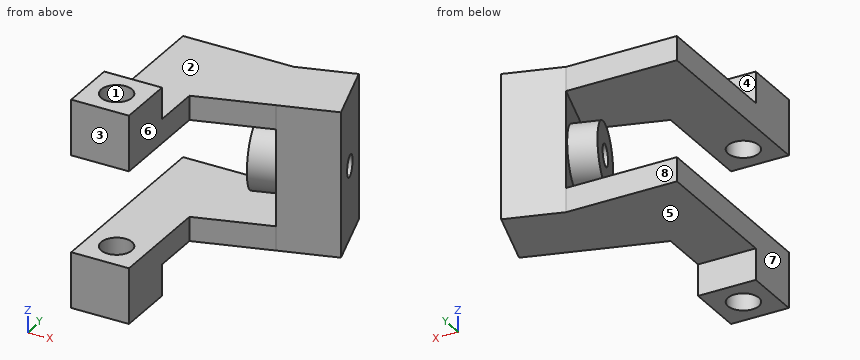
from build123d import *

# Parameters (mm, degrees)
BOSS_EXTRUDE1_DEPTH     = 9.525
SKETCH2_W               = 12.7
SKETCH2_H               = 25.806397913
CUT_EXTRUDE1_DEPTH      = 14.822389654
CUT_EXTRUDE1_DEPTH_BACK = 4.513666667
SKETCH3_W               = 19.05
SKETCH3_H               = 9.271
SKETCH3_R               = 1.397
BOSS_EXTRUDE2_DEPTH     = 7.62
SKETCH3_3_R             = 4.064
SKETCH3_3_R_2           = 1.397
BOSS_EXTRUDE3_DEPTH     = 3.556
SKETCH4_W               = 4.1275
SKETCH4_H               = 7.62
BOSS_EXTRUDE4_DEPTH     = 7.62
SKETCH5_R               = 2.032
CUT_EXTRUDE2_DEPTH      = 20.0025


with BuildPart() as part:
    # Sketch1 → Boss-Extrude1 (new body, symmetric)
    with BuildSketch(Plane.XY):
        Polygon((-3.513666667, -7.641166667), (4.106333333, -7.641166667), (4.106333333, 6.328833333), (13.822389654, 9.299329853), (11.111811579, 18.165231246), (-3.513666667, 18.165231246), align=None)
    extrude(amount=BOSS_EXTRUDE1_DEPTH, both=True)

    # Sketch2 → Cut-Extrude1 (cut, two sides)
    with BuildSketch(Plane(origin=(0, 0, 0), x_dir=(0, 0, -1), z_dir=(1, 0, 0))) as cut_extrude1_sk:
        with Locations((0, 5.26203229)):
            Rectangle(SKETCH2_W, SKETCH2_H)
    extrude(amount=CUT_EXTRUDE1_DEPTH, mode=Mode.SUBTRACT)
    extrude(cut_extrude1_sk.sketch, amount=-CUT_EXTRUDE1_DEPTH_BACK, mode=Mode.SUBTRACT)

    # Sketch3 → Boss-Extrude2 (add)
    with BuildSketch(Plane(origin=(15.24089464, 4.659609104, 0), x_dir=(0, 0, -1), z_dir=(0.956304756, 0.292371705, 0))):
        with Locations((0, 9.48721774)):
            Rectangle(SKETCH3_W, SKETCH3_H)
        with Locations((0, 9.48721774)):
            Circle(SKETCH3_R, mode=Mode.SUBTRACT)
    extrude(amount=BOSS_EXTRUDE2_DEPTH)

    # Sketch3<3> → Boss-Extrude3 (add)
    with BuildSketch(Plane(origin=(15.24089464, 4.659609104, 0), x_dir=(0, 0, -1), z_dir=(0.956304756, 0.292371705, 0))):
        with Locations((0, 9.48721774)):
            Circle(SKETCH3_3_R)
        with Locations((0, 9.48721774)):
            Circle(SKETCH3_3_R_2, mode=Mode.SUBTRACT)
    extrude(amount=-BOSS_EXTRUDE3_DEPTH)

    # Sketch4 → Boss-Extrude4 (add)
    with BuildSketch(Plane(origin=(4.106333333, 0, 0), x_dir=(0, 0, -1), z_dir=(1, 0, 0))):
        with Locations((-11.58875, -3.831166667)):
            Rectangle(SKETCH4_W, SKETCH4_H)
    boss_extrude4 = extrude(amount=-BOSS_EXTRUDE4_DEPTH)

    # Sketch5 → Cut-Extrude2 (cut)
    with BuildSketch(Plane.XY.offset(13.6525)):
        with Locations((0.296333333, -3.831166667)):
            Circle(SKETCH5_R)
    cut_extrude2 = extrude(amount=-CUT_EXTRUDE2_DEPTH, mode=Mode.SUBTRACT)

    # Mirror1: Boss-Extrude4, Cut-Extrude2 across plane
    add(boss_extrude4.mirror(Plane.XY))
    add(cut_extrude2.mirror(Plane.XY), mode=Mode.SUBTRACT)


solid = part.part
Geometry check sheet. Reference: the model listing, model coordinates, mm. Face numbers are marked on the shaded views. A direction names the side the tool comes from. Give positions to 0.01 mm unless a question says otherwise; leave off trailing zeros. Order: outer loops, then holes, each group sorted by start corner. A loop starts at its lowest first (then second) coordinate and runs counter-clockwise, first axis right, second up.
1. Sectioned sample at D-D (y = 5.5). Record the boundary of the cut face in (x, z) (3 decimals), then the cut area to 3 significant figures.
Completed:
outline: (-3.514, -9.525) - (4.106, -9.525) - (4.106, -6.35) - (-3.514, -6.35) - close; (-3.514, 6.35) - (4.106, 6.35) - (4.106, 9.525) - (-3.514, 9.525) - close
area: 48.4 mm2
2. Draft check along Y on the marked faces 1, 2 and 3. Enter one of: pulls with the +Y half, pulls with the -Y half, needs draft (parallel to the pull), parting line crosses it, or undercut.
Completed:
face 1: undercut
face 2: needs draft
face 3: pulls with the -Y half
3. Sectioned sample at C-C (y = -5). Record the boundary of the cut face in (x, z), then the cut area to 3 significant figures.
Completed:
outline: (-3.51, -13.65) - (-1.37, -13.65) - (-1.37, -6.35) - (-3.51, -6.35) - close; (-3.51, 6.35) - (-1.37, 6.35) - (-1.37, 13.65) - (-3.51, 13.65) - close; (1.96, -13.65) - (4.11, -13.65) - (4.11, -6.35) - (1.96, -6.35) - close; (1.96, 6.35) - (4.11, 6.35) - (4.11, 13.65) - (1.96, 13.65) - close
area: 62.7 mm2
4. Depth check by flat-ended pin: pin 1 (3 mm diameter, centred on x = 1, y = 4.5, fed in from +Z) (3 decimals); pin 2 (2.5 mm diameter, centred on x = 5.5, z = 7.5, fed in from +Y); pin 3 (1.5 mm diameter, centred on x = 6, z = -7, fed in from -Y). Enter the tip coordinate at first touch or a pass-through.
Completed:
pin 1: stops at z = 9.525
pin 2: stops at y = 18.17
pin 3: stops at y = 6.68
5. Sectioned sample at A-A (y = -0.75). Record the boundary of the cut face in (x, z).
Completed:
outline: (-3.51, -13.65) - (4.11, -13.65) - (4.11, -6.35) - (-3.51, -6.35) - close; (-3.51, 6.35) - (4.11, 6.35) - (4.11, 13.65) - (-3.51, 13.65) - close
6. Sectioned sample at B-B (z = 3.5). Record the boundary of the cut face in (x, y).
Completed:
outline: (8.46, 14.67) - (9.67, 10.72) - (13.07, 11.76) - (13.82, 9.3) - (21.11, 11.53) - (18.4, 20.39) - (11.11, 18.17) - (11.86, 15.71) - close
7. Access from +Z, -Z, +X, -X, +Y, -Y to the whole of each face (thin tool, end or side, straight path). Record for the marked faces 4, 5, 6, 7 and 8.
Completed:
face 4: +Z, +X, -X, +Y
face 5: -Z, +X, -X, +Y
face 6: +Z, -Z, +X, -Y
face 7: +Z, -Z, -X, +Y, -Y
face 8: +Z, -Z, -X, +Y
8. Scan lines: line 1 (Z direction, x = 5, y = 10.75) (3 decimals); line 2 (Z direction, x = 10.5, y = 14.25) (3 decimals); line 3 (Z direction, x = 11, y = 13) (3 decimals). Record each from-to range of solid material in increasing order.
Completed:
line 1: z = -9.525 to -6.35, 6.35 to 9.525
line 2: z = -9.525 to -6.35, -3.921 to -0.898, 0.898 to 3.921, 6.35 to 9.525
line 3: z = -9.525 to -6.35, -4.055 to -1.37, 1.37 to 4.055, 6.35 to 9.525
